The model under review builds one solid part; all positions refer to its coordinate system, in mm. Coordinates: 2 decimals unless noted, no trailing zeros. Write each loop counter-clockwise with the first axis right and the second up, starting at its lowest first coordinate (ties: lowest second). Pieces come first, ordered by that corner, then holes. Notation, with made-up numbers: (44.5, 2.25) - (79.5, 2.25) arc R12 ccw to (79.5, 11.25) - close; hole circle Ø7 at (-26, 30.5). An arc over 180 degrees is marked (long way). Return JSON: item names as keys, results as strings. Group by question number.
(1) Draft analysis for pull direction Z (two halves, no side actions). For faces 1 (the face through (62, 1, -26.361)), 2 (the face through (79.78, 1.52, -18.21)), 3 (the face through (-8.625, 1, -18)), state which applies: released by +Z, released by -Z, zero draft, split by the parting line, or undercut.
(2) We need section B-B on y = 1.35. State the section outline as (x, z) points, then the cut area to 3 significant figures.
(3) For pin 1 Ø2.5 at (x, z) = (81.11, -18.9) entering from -Y, flat-tipped, find the tip position at first contact; note if it passes through.
(4) We need section A-A on z = -19. State the section outline as (x, y) points.
(5) To check wall thickness, follow L1, parallel to X at y = 1.1, z = -18.75; L2, parallel to Z at x = 40, y = 2.4; L3, parallel to X at y = 1, z = -24. State the ranges of each line that lie inside material, in increasing order. Write a range as from..to.
```python
from build123d import *

# Parameters (mm, degrees)
BOSS_EXTRUDE1_DEPTH = 3
CUT_EXTRUDE1_REACH  = 136.027
SKETCH4_R           = 1.5


with BuildPart() as part:
    # Sketch3 → Boss-Extrude1 (new body)
    with BuildSketch(Plane(origin=(0, 0, 0), x_dir=(1, 0, 0), z_dir=(0, 1, 0))):
        with BuildLine():
            Line((125.49028015, 26.360794257), (-2.74094445, 26.360794257))
            ThreePointArc((-2.74094445, 26.360794257), (-3.945556452, 25.430743303), (-5.431022837, 25.099874039))
            Line((-5.431022837, 25.099874039), (-5.62533215, 25.099874039))
            ThreePointArc((-5.62533215, 25.099874039), (-7.746652493, 24.221194382), (-8.62533215, 22.099874039))
            Line((-8.62533215, 22.099874039), (-8.62533215, 14.358894177))
            Line((-8.62533215, 14.358894177), (131.37466785, 14.358894177))
            Line((131.37466785, 14.358894177), (131.37466785, 22.099874039))
            ThreePointArc((131.37466785, 22.099874039), (130.495988194, 24.221194382), (128.37466785, 25.099874039))
            Line((128.37466785, 25.099874039), (128.180358538, 25.099874039))
            ThreePointArc((128.180358538, 25.099874039), (126.694892152, 25.430743303), (125.49028015, 26.360794257))
        make_face()
    extrude(amount=BOSS_EXTRUDE1_DEPTH)

    # Sketch4 → Cut-Extrude1 (cut, up to next)
    with BuildSketch(Plane(origin=(0, 3, 0), x_dir=(1, 0, 0), z_dir=(0, 1, 0)), mode=Mode.PRIVATE) as cut_extrude1_sk1:
        with Locations(Location((81.109797099, 18.903114067, 0), (0, 0, 270))):
            Circle(SKETCH4_R)
    cut_extrude1_tool1 = extrude(cut_extrude1_sk1.sketch, amount=-CUT_EXTRUDE1_REACH, mode=Mode.PRIVATE) & part.part
    # Sketch4 → Cut-Extrude1 (cut, up to next)
    with BuildSketch(Plane(origin=(0, 3, 0), x_dir=(1, 0, 0), z_dir=(0, 1, 0)), mode=Mode.PRIVATE) as cut_extrude1_sk2:
        with BuildLine():
            ThreePointArc((41.109797099, 20.503114067), (39.509797099, 18.903114067), (41.109797099, 17.303114067))
            ThreePointArc((41.109797099, 17.303114067), (42.709797099, 18.903114067), (41.109797099, 20.503114067))
        make_face()
    cut_extrude1_tool2 = extrude(cut_extrude1_sk2.sketch, amount=-CUT_EXTRUDE1_REACH, mode=Mode.PRIVATE) & part.part
    add(cut_extrude1_tool1.solids().sort_by_distance((81.109797, 3, -18.903114))[0], mode=Mode.SUBTRACT)
    add(cut_extrude1_tool2.solids().sort_by_distance((41.109797, 3, -18.903114))[0], mode=Mode.SUBTRACT)


solid = part.part
```
Ans:
{
 "1": {"face 1": "released by -Z", "face 2": "undercut", "face 3": "zero draft"},
 "2": {"outline": "(-8.63, -22.1) arc R3 ccw to (-5.63, -25.1) - (-5.43, -25.1) arc R3.5 cw to (-2.74, -26.36) - (125.49, -26.36) arc R3.5 cw to (128.18, -25.1) - (128.37, -25.1) arc R3 ccw to (131.37, -22.1) - (131.37, -14.36) - (-8.63, -14.36) - close; hole circle Ø3.2 at (41.11, -18.9); hole circle Ø3 at (81.11, -18.9)", "area": "1,650 mm²"},
 "3": {"pin 1": "through"},
 "4": {"outline": "(-8.63, 0) - (39.51, 0) - (39.51, 3) - (-8.63, 3) - close; (42.71, 0) - (79.61, 0) - (79.61, 3) - (42.71, 3) - close; (82.61, 0) - (131.37, 0) - (131.37, 3) - (82.61, 3) - close"},
 "5": {"L1": "-8.63..39.52, 42.7..79.62, 82.6..131.37", "L2": "-26.36..-20.06, -17.75..-14.36", "L3": "-7.95..130.7"}
}
